Geometry: see drawing. Coordinates: mm, zero at the bounding-box minimum. A direction names the side the tool comes from. Give positions to 0.01 mm unless a question says otherwise; leave off trailing zeros. Order: outer loops, then holes, each group sorted by start corner. A loop starts at its lowest first (then second) coordinate and runs counter-clockwise, first axis right, second up. Notation, with made-up numbers: M 24,26.25 L 45,26.25 A7 ccw 45,34.25 Z; hole C 54.25,-25 d9. An arc over 180 degrees is marked long. Use a Markdown table: item, result.
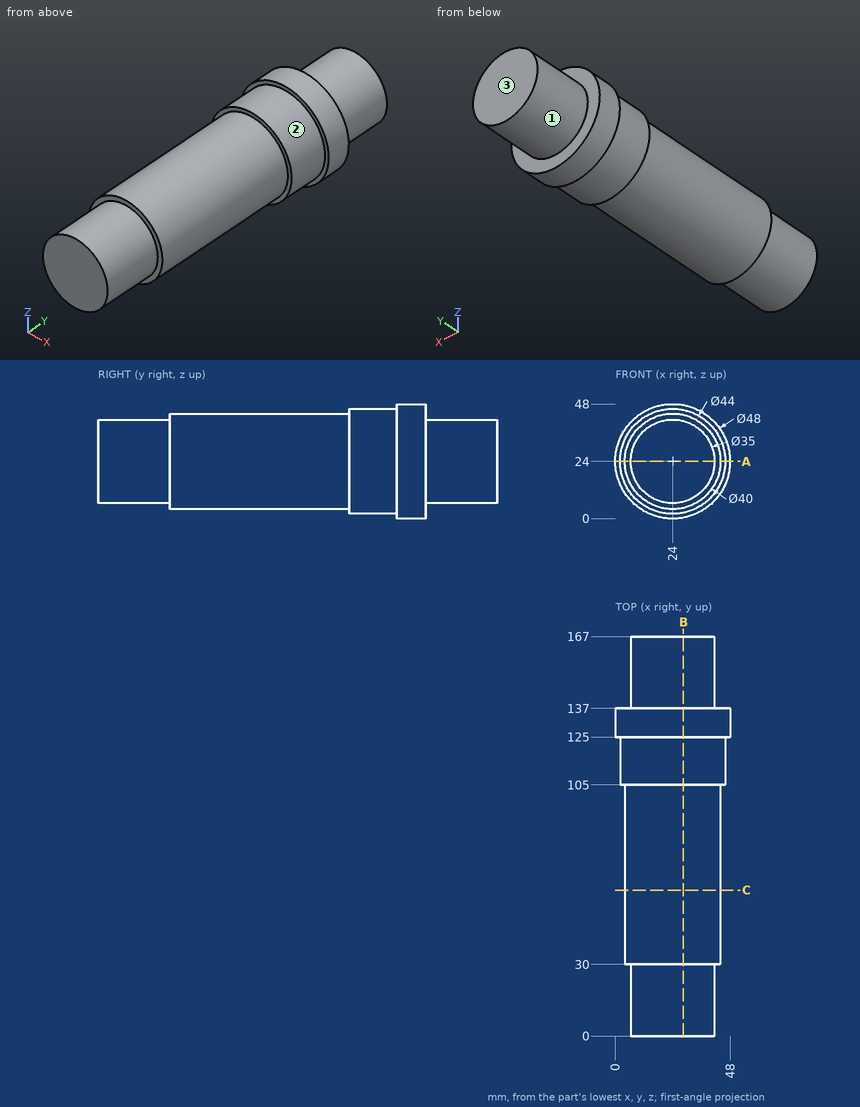
1) Cut plane B-B on x = 28.5. Return loops of the section in (y, z).
Response values:
| item | result |
|---|---|
| outline | M 0,7.09 L 30,7.09 L 30,4.51 L 105,4.51 L 105,2.47 L 125,2.47 L 125,0.43 L 137,0.43 L 137,7.09 L 167,7.09 L 167,40.91 L 137,40.91 L 137,47.57 L 125,47.57 L 125,45.53 L 105,45.53 L 105,43.49 L 30,43.49 L 30,40.91 L 0,40.91 Z |
2) Material intervals for line 1 (Y direction, x = 4.5, z = 23.5); line 2 (Z direction, x = 23, y = 109); line 3 (Y direction, x = 12, z = 40.5), sorted ascending. Write a range as from..to.
Response values:
| item | result |
|---|---|
| line 1 | y = 30..137 |
| line 2 | z = 2.02..45.98 |
| line 3 | y = 105..137 |
3) Cut plane A-A on z = 24. Return loops of the section in (x, y).
Response values:
| item | result |
|---|---|
| outline | M 0,125 L 2,125 L 2,105 L 4,105 L 4,30 L 6.5,30 L 6.5,0 L 41.5,0 L 41.5,30 L 44,30 L 44,105 L 46,105 L 46,125 L 48,125 L 48,137 L 41.5,137 L 41.5,167 L 6.5,167 L 6.5,137 L 0,137 Z |
4) First-contact query: pin 1 Ø1 at (x, y) = (26.5, 138.5) entering from -Z; pin 2 Ø1.5 at (y, z) = (94, 21.5) entering from +X; pin 3 Ø3 at (x, z) = (9.5, 7.5) entering from -Y. Flat tips, straight axial feed; report the tip coordinate or a pass-through.
Response values:
| item | result |
|---|---|
| pin 1 | stops at z = 6.61 |
| pin 2 | stops at x = 43.92 |
| pin 3 | stops at y = 105 |
5) Reachability of the marked faces 1, 2 and 3 from +Z, -Z, +X, -X, +Y, -Y: full face, straight path, thin tool, end or side. Return the list, or none.
Response values:
| item | result |
|---|---|
| face 1 | +Y |
| face 2 | -Y |
| face 3 | +Z, -Z, +X, -X, +Y |
6) Cut plane C-C on y = 61. Return loops of the section in (x, z).
Response values:
| item | result |
|---|---|
| outline | C 24,24 d40 |
